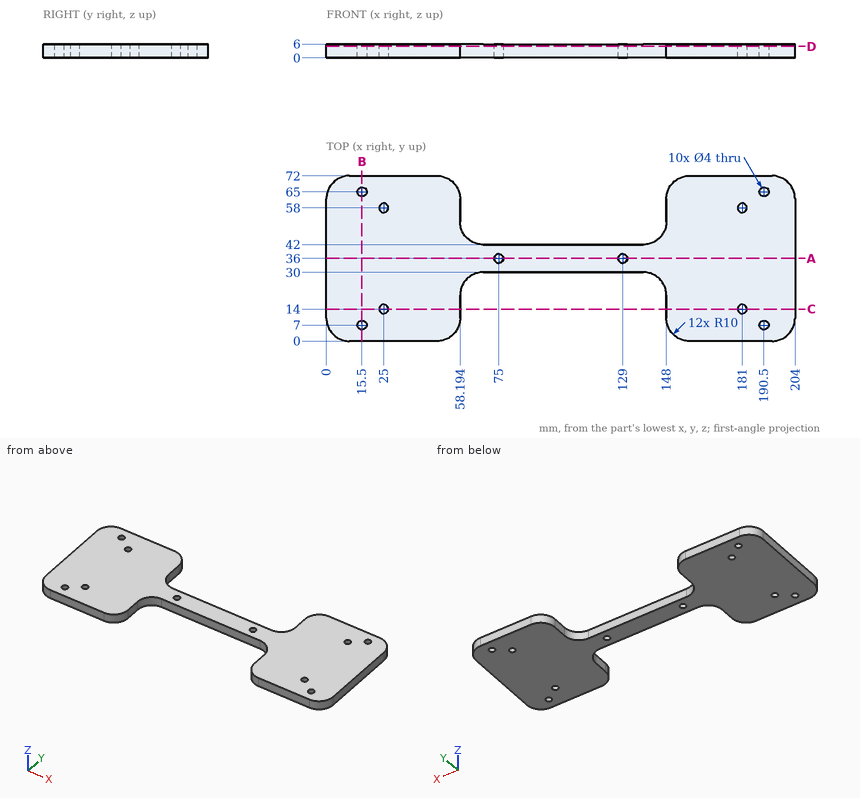
Input: dimensioned drawing with shaded views. Units: mm. Origin: part minimum x, y, z. Coordinates: 2 decimals unless noted, no trailing zeros. Loops run counter-clockwise (first coordinate to the right, second up) from the corner with the lowest first, then second, coordinate; pieces in that order, holes last. Notation, with made-up numbers: M 74.5,53 L 122.5,53 A34 ccw 122.5,83 Z; hole C 17.5,4.5 d4. An arc over 180 degrees is marked long. One line per item, written item: value. Start each with the question number.
1) Cut plane C-C (y = 14). Return loops of the section in (x, z) (1 decimal), then the cut area to 3 significant figures.
2) Material intervals for L1, parallel to Y at x = 15.5, z = 2.7; L2, parallel to Y at x = 25, z = 2.05; L3, parallel to X at y = 36, z = 4.6, sorted ascending. Write a range as from..to.
3) Cut plane A-A (y = 36). Return loops of the section in (x, z).
4) Pin query (flat end, axial travel): P1, Ø2.5, axis at x = 181, y = 14, coming from the -Z side; P2, Ø1.8, axis at x = 87, z = 4.5, coming from the +Y side; P3, Ø1.8, axis at x = 106.5, z = 3, coming from the -Y side; P4, Ø2, axis at x = 52, z = 1, coming from the -Y side. Return the tip coordinate at first contact, or that it passes through.
5) Cut plane D-D (z = 5). Count the separate pieces of the cut face and the enclosed holes in it, then the cut area to 3 significant figures.
6) Cut plane B-B (x = 15.5). Return loops of the section in (y, z), then the cut area to 3 significant figures.
Evaluation:
1. outline: M 0,0 L 23,0 L 23,6 L 0,6 Z; M 27,0 L 58.2,0 L 58.2,6 L 27,6 Z; M 148,0 L 179,0 L 179,6 L 148,6 Z; M 183,0 L 204,0 L 204,6 L 183,6 Z
1. area: 637 mm^2
2. L1: 0..5, 9..63, 67..72
2. L2: 0..12, 16..56, 60..72
2. L3: 0..73, 77..127, 131..204
3. outline: M 0,0 L 73,0 L 73,6 L 0,6 Z; M 77,0 L 127,0 L 127,6 L 77,6 Z; M 131,0 L 204,0 L 204,6 L 131,6 Z
4. P1: through
4. P2: y = 42
4. P3: y = 30
4. P4: y = 0.4
5. separate pieces: 1
5. enclosed holes: 10
5. area: 9,090 mm^2
6. outline: M 0,0 L 5,0 L 5,6 L 0,6 Z; M 9,0 L 63,0 L 63,6 L 9,6 Z; M 67,0 L 72,0 L 72,6 L 67,6 Z
6. area: 384 mm^2
